```python
from build123d import *

# Parameters (mm, degrees)
CYLINDER006_R     = 17.5
CYLINDER006_DEPTH = 10
CYLINDER005_R     = 22.5
CYLINDER005_DEPTH = 5


with BuildPart() as cylinder006:
    # Cylinder006 → Cylinder006 (new body)
    with BuildSketch(Plane.XY):
        Circle(CYLINDER006_R)
    extrude(amount=CYLINDER006_DEPTH)


with BuildPart() as cut005:
    # Cylinder005 → Cylinder005 (new body)
    with BuildSketch(Plane.XY):
        Circle(CYLINDER005_R)
    extrude(amount=CYLINDER005_DEPTH)

    # Cut005: cut Cylinder006
    add(cylinder006.part, mode=Mode.SUBTRACT)


solid = cut005.part
```
Source: CAD feature listing. Evaluate the final solid. Frame: model axes, mm. Coordinates: 2 decimals unless noted, no trailing zeros. Order: outer loops, then holes, each group sorted by start corner. A loop starts at its lowest first (then second) coordinate and runs counter-clockwise, first axis right, second up. Notation, with made-up numbers: M -39,31.5 L -24,31.5 A32 ccw -24,61.5 Z; hole C -19.5,89 d7. An arc over 180 degrees is marked long. Write each question's results on one line, items separated by ' | '. Start each with the question number.
1) Draft query along Y for faces 1 (the face through (10.382, -19.961, 2.465)), 2 (the face through (-13.887, -10.648, 2.465)), 3 (the face through (12, -13, 5)). Return one class per face: released by +Y, released by -Y, zero draft, split by the parting line, or undercut.
2) Contact query for flat-ended pins moving along their axis: pin 1 Ø21 at (x, y) = (0, 0) entering from -Z; pin 2 Ø1.5 at (x, z) = (-9.5, 2.5) entering from +Y; pin 3 Ø2 at (x, z) = (-12, 2.5) entering from +Y. Output: stop coordinate, or through.
3) Line query: line 1 (Y direction, x = 0, z = 3.7); line 2 (Y direction, x = -12, z = 0.7); line 3 (X direction, y = -9, z = 3.95). Output: solid intervals per line, ascending. Write a range as from..to.
4) Section query A-A (x = 0). Return the cut outline in (y, z), plus the area to 3 significant figures.
5) Section query C-C (z = 4.45). Return the cut outline in (x, y), plus the area to 3 significant figures.
Answers:
1) face 1: split by the parting line | face 2: undercut | face 3: zero draft
2) pin 1: passes through | pin 2: stops at y = 20.73 | pin 3: stops at y = 19.63
3) line 1: y = -22.5..-17.5, 17.5..22.5 | line 2: y = -19.03..-12.74, 12.74..19.03 | line 3: x = -20.62..-15.01, 15.01..20.62
4) outline: M -22.5,0 L -17.5,0 L -17.5,5 L -22.5,5 Z; M 17.5,0 L 22.5,0 L 22.5,5 L 17.5,5 Z | area: 50.0 mm^2
5) outline: C 0,0 d45; hole C 0,0 d35 | area: 628 mm^2
